Build history of the part. All positions in model axes, mm. Give positions to 0.01 mm unless a question says otherwise; leave off trailing zeros. Loops run counter-clockwise (first coordinate to the right, second up) from the corner with the lowest first, then second, coordinate; pieces in that order, holes last. Notation, with made-up numbers: (-14, 15.5) -> (8, 15.5) arc R25 cw to (8, 53.5) -> close; hole circle Ø7 at (25.5, -19.5). An arc over 180 degrees is marked (long way). Answer as a JSON object with one key per item and string values. Group by question number.
Q1. Wall check: probe 1 along X at (y, z) = (2, 0.55); probe 2 along Y at (x, z) = (2, 0.85); probe 3 along X at (y, z) = (26, 0.2). Give the ranges that are in metal, low to high. Write a range as from..to.
Q2. Band-saw the part on B-B, the plane x = 2. Write the cut outline in (y, z), plus the area to 3 significant figures.
Q3. Band-saw the part on C-C, the plane y = 2. Write the cut outline in (x, z), plus the area to 3 significant figures.
Q4. Band-saw the part on A-A, the plane z = 0.85. Write the cut outline in (x, y), plus the area to 3 significant figures.
Autodesk Inventor part; units mm, degrees
ref_plane "YZ Plane" through (0, 0, 0) normal (1, 0, 0) x (0, 1, 0)
ref_plane "XZ Plane" through (0, 0, 0) normal (0, 1, 0) x (-1, 0, 0)
ref_plane "XY Plane" through (0, 0, 0) normal (0, 0, 1) x (1, 0, 0)
sketch "Sketch1" plane through (0, 0, 0) normal (0, 0, 1) x (1, 0, 0)
  line L0 (0, 0) -> (31.4, 0)
  line L1 (31.4, 0) -> (31.4, 27.4)
  line L2 (31.4, 27.4) -> (0, 27.4)
  line L3 (0, 27.4) -> (0, 0)
  dimension "d0" = 31.4
  dimension "d1" = 27.4
extrude "Extrusion1" add sketch "Sketch1" along normal blind 1
sketch "Sketch17" plane through (0, 0, 1) normal (0, 0, 1) x (1, 0, 0)
  line L0 (2, 25.4) -> (29.4, 25.4) construction
  line L1 (29.4, 25.4) -> (29.4, 2) construction
  line L2 (29.4, 2) -> (2, 2) construction
  line L3 (2, 2) -> (2, 25.4) construction
  line L4 (0, 0) -> (0, 27.4) construction
  line L5 (0, 27.4) -> (31.4, 27.4) construction
  dimension "d169" = 27.4
  dimension "d170" = 23.4
  dimension "d171" = 2
  dimension "d172" = 2
hole "Hole16" at (2, 25.4, 1) at (29.4, 25.4, 1) at (29.4, 2, 1) at (2, 2, 1) direction (0, 0, -1) diameter 2.3 end through all
properties part number "Mixer IQ Box ND20" material "Aluminum-6061"
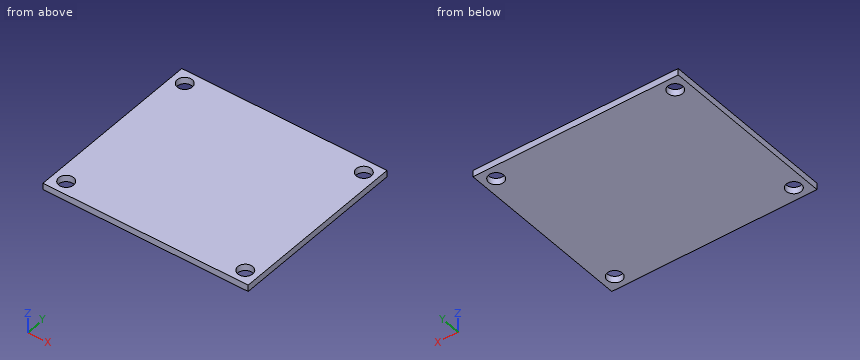
Worked answers:
{
 "1": {"probe 1": "0..0.85, 3.15..28.25, 30.55..31.4", "probe 2": "0..0.85, 3.15..24.25, 26.55..27.4", "probe 3": "0..1.02, 2.98..28.42, 30.38..31.4"},
 "2": {"outline": "(0, 0) -> (0.85, 0) -> (0.85, 1) -> (0, 1) -> close; (3.15, 0) -> (24.25, 0) -> (24.25, 1) -> (3.15, 1) -> close; (26.55, 0) -> (27.4, 0) -> (27.4, 1) -> (26.55, 1) -> close", "area": "22.8 mm2"},
 "3": {"outline": "(0, 0) -> (0.85, 0) -> (0.85, 1) -> (0, 1) -> close; (3.15, 0) -> (28.25, 0) -> (28.25, 1) -> (3.15, 1) -> close; (30.55, 0) -> (31.4, 0) -> (31.4, 1) -> (30.55, 1) -> close", "area": "26.8 mm2"},
 "4": {"outline": "(0, 0) -> (31.4, 0) -> (31.4, 27.4) -> (0, 27.4) -> close; hole circle Ø2.3 at (2, 2); hole circle Ø2.3 at (2, 25.4); hole circle Ø2.3 at (29.4, 2); hole circle Ø2.3 at (29.4, 25.4)", "area": "844 mm2"}
}
